Read the model definition and answer for the solid it produces. Units are mm, in the model's axes. Face numbers are marked on the shaded views. A direction names the side the tool comes from. Give positions to 0.01 mm unless a question says otherwise; leave off trailing zeros. Loops run counter-clockwise (first coordinate to the right, second up) from the corner with the lowest first, then second, coordinate; pieces in that order, holes last. Notation, with made-up numbers: (-14, 8) - (19, 8) arc R38 cw to (19, 46) - close; hole circle Ø5 at (69, 69). An arc over 180 degrees is marked (long way). Use a Markdown table: item, result. Add a question column.
Item 1: Consider probe 1 along Y at (x, z) = (0.5, 1); probe 2 along Y at (x, z) = (-0.25, -2.5); probe 3 along Z at (x, y) = (0, -9.75). Determine where each line is inside the solid, lowest interval first. Write a range as [from, to].
Item 2: For a pull along X with two mould halves and no side action, classify the marked faces 1, 2 and 3 as +X half, -X half, draft (parallel to the pull), parting line (faces both ways), or undercut.
Item 3: Each of these flat-tipped pins is pushed along its axis until it touches: P1, Ø2, axis at x = -0.5, z = -0.5, coming from the +Y side; P2, Ø3, axis at x = 2, y = -3, coming from the -Z side. Where does it stop, or does it pass through?
Item 4: Which of the six approach directions +Z, -Z, +X, -X, +Y, -Y give full straight-line access (tool end or side, diameter ignored) to the marked faces 4, 5 and 6?
Item 5: A cutting plane is placed at B-B (y = -4.75). Determine the outline of the cut face in (x, z), plus the area to 3 significant figures.
Item 6: A cutting plane is placed at A-A (x = 0). Determine the outline of the cut face in (y, z).
Autodesk Inventor part; units mm, degrees
ref_plane "YZ Plane" through (0, 0, 0) normal (1, 0, 0) x (0, 1, 0)
ref_plane "XZ Plane" through (0, 0, 0) normal (0, 1, 0) x (-1, 0, 0)
ref_plane "XY Plane" through (0, 0, 0) normal (0, 0, 1) x (1, 0, 0)
sketch "Sketch1" plane through (0, 0, 0) normal (0, 1, 0) x (-1, 0, 0)
  circle A0 centre (0, 0) radius 3
  dimension "d0" = 6
extrude "Extrusion1" add sketch "Sketch1" against normal blind 3
sketch "Sketch2" plane through (0, -3, 0) normal (0, -1, 0) x (1, 0, 0)
  circle A0 centre (0, 0) radius 1.5
  dimension "d3" = 3
extrude "Extrusion2" add sketch "Sketch2" along normal blind 8
sketch "Sketch3" plane through (0, 0, 0) normal (0, 1, 0) x (1, 0, 0)
  circle A0 centre (0, 0) radius 1.5 construction
  line L0 (1.4434, 0) -> (0.7217, -1.25)
  line L1 (0.7217, -1.25) -> (-0.7217, -1.25)
  line L2 (-0.7217, -1.25) -> (-1.4434, 0)
  line L3 (-1.4434, 0) -> (-0.7217, 1.25)
  line L4 (-0.7217, 1.25) -> (0.7217, 1.25)
  line L5 (0.7217, 1.25) -> (1.4434, 0)
  dimension "d8" = 2.5
extrude "Extrusion3" cut sketch "Sketch3" against normal blind 1.5
chamfer "Chamfer1" distance 0.25 angle 45 1 edges at (-1.5, -11, 0)
fillet "Fillet1" radius 0.25 2 edges at (3, 0, 0) (3, -3, 0)
chamfer "Chamfer2" distance 0.1 angle 45 6 edges at (0, 0, -1.25) (1.0825, 0, -0.625) (1.0825, 0, 0.625) (0, 0, 1.25) (-1.0825, 0, 0.625) (-1.0825, 0, -0.625)
thread "Thread2"
properties part number "M3-8" material "Steel, Carbon"
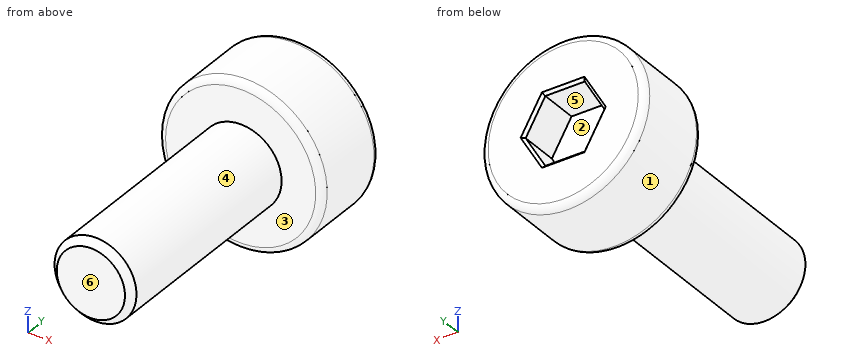
Geometry says:
| question | item | result |
|---|---|---|
| 1 | probe 1 | [-11, -1.5] |
| 1 | probe 2 | [-3, 0] |
| 1 | probe 3 | [-1.5, 1.5] |
| 2 | face 1 | parting line |
| 2 | face 2 | undercut |
| 2 | face 3 | draft |
| 3 | P1 | y = 0 |
| 3 | P2 | z = -2.95 |
| 4 | face 4 | -Y |
| 4 | face 5 | +Y |
| 4 | face 6 | +Z, -Z, +X, -X, -Y |
| 5 | outline | circle Ø3 at (0, 0) |
| 5 | area | 7.07 mm² |
| 6 | outline | (-11, -1.25) - (-10.75, -1.5) - (-3, -1.5) - (-3, -2.75) arc R0.25 ccw to (-2.75, -3) - (-0.25, -3) arc R0.25 ccw to (0, -2.75) - (0, -1.35) - (-0.1, -1.25) - (-1.5, -1.25) - (-1.5, 1.25) - (-0.1, 1.25) - (0, 1.35) - (0, 2.75) arc R0.25 ccw to (-0.25, 3) - (-2.75, 3) arc R0.25 ccw to (-3, 2.75) - (-3, 1.5) - (-10.75, 1.5) - (-11, 1.25) - close |
